from build123d import *

# Parameters (mm, degrees)
SKETCH1_R                 = 3.35
BOSS_EXTRUDE1_DEPTH       = 2.7
SKETCH2_R                 = 2.4
BOSS_EXTRUDE2_DEPTH       = 1.4
SKETCH3_R                 = 1.95
BOSS_EXTRUDE3_DEPTH       = 0.5
F_2_0MM_DOWEL_HOLE1_D     = 2
F_2_0MM_DOWEL_HOLE1_DEPTH = 52.32
F_2_0MM_DOWEL_HOLE1_TIP   = 0.600860619
SKETCH7_W                 = 5.275172559
SKETCH7_H                 = 2.8
BOSS_EXTRUDE4_DEPTH       = 2
F_2_0MM_DOWEL_HOLE2_D     = 1.2
F_2_0MM_DOWEL_HOLE2_DEPTH = 52.32
F_2_0MM_DOWEL_HOLE2_TIP   = 0.360516371
BOSS_EXTRUDE5_DEPTH       = 2.3
BOSS_EXTRUDE6_DEPTH       = 0.5
LPATTERN1_COUNT           = 2
LPATTERN1_PITCH           = 3.5
SKETCH12_R                = 0.5
BOSS_EXTRUDE7_DEPTH       = 1
SKETCH13_W                = 0.512018779
SKETCH13_H                = 0.9
BOSS_EXTRUDE8_DEPTH       = 0.6
BOSS_EXTRUDE9_DEPTH       = 4
SKETCH6_R                 = 2.1
CUT_EXTRUDE1_DEPTH        = 2
SKETCH17_R                = 0.625
CUT_EXTRUDE2_DEPTH        = 2
FILLET1_R                 = 0.1
FILLET2_R                 = 2.7
FILLET3_R                 = 0.5
SKETCH18_R                = 2.8
CUT_EXTRUDE3_DEPTH        = 0.8
BOSS_EXTRUDE10_START      = 0.8
BOSS_EXTRUDE10_DEPTH      = 0.8


with BuildPart() as part:
    # Sketch1 → Boss-Extrude1 (new body)
    with BuildSketch(Plane.XY):
        with Locations(Location((0, 0, 0), (0, 0, 180))):
            Circle(SKETCH1_R)
    extrude(amount=BOSS_EXTRUDE1_DEPTH)

    # Sketch2 → Boss-Extrude2 (add)
    with BuildSketch(Plane.XY.offset(2.7)):
        Circle(SKETCH2_R)
    extrude(amount=BOSS_EXTRUDE2_DEPTH)

    # Sketch3 → Boss-Extrude3 (add)
    with BuildSketch(Plane.XY.offset(4.1)):
        Circle(SKETCH3_R)
    extrude(amount=BOSS_EXTRUDE3_DEPTH)

    # Ø2.0mm Dowel Hole1
    with Locations(Plane.XY.offset(4.6)):
        with Locations((0, 0)):
            Hole(F_2_0MM_DOWEL_HOLE1_D / 2, depth=F_2_0MM_DOWEL_HOLE1_DEPTH)
            with Locations((0, 0, -(F_2_0MM_DOWEL_HOLE1_DEPTH + F_2_0MM_DOWEL_HOLE1_TIP / 2))):  # 118° drill point
                Cone(0, F_2_0MM_DOWEL_HOLE1_D / 2, F_2_0MM_DOWEL_HOLE1_TIP, mode=Mode.SUBTRACT)

    # Sketch7 → Boss-Extrude4 (add)
    with BuildSketch(Plane(origin=(0, 0, 0.4), x_dir=(-1, 0, 0), z_dir=(0, 0, -1))):
        with Locations((4.812413721, 1.05)):
            Rectangle(SKETCH7_W, SKETCH7_H)
    extrude(amount=-BOSS_EXTRUDE4_DEPTH)

    # Ø2.0mm Dowel Hole2
    with Locations(Plane(origin=(0, 0, 0.4), x_dir=(-1, 0, 0), z_dir=(0, 0, -1))):
        with Locations((5.95, 1.35)):
            Hole(F_2_0MM_DOWEL_HOLE2_D / 2, depth=F_2_0MM_DOWEL_HOLE2_DEPTH)
            with Locations((0, 0, -(F_2_0MM_DOWEL_HOLE2_DEPTH + F_2_0MM_DOWEL_HOLE2_TIP / 2))):  # 118° drill point
                Cone(0, F_2_0MM_DOWEL_HOLE2_D / 2, F_2_0MM_DOWEL_HOLE2_TIP, mode=Mode.SUBTRACT)

    # Sketch10 → Boss-Extrude5 (add)
    with BuildSketch(Plane(origin=(0, 0, 0.4), x_dir=(-1, 0, 0), z_dir=(0, 0, -1))):
        with BuildLine():
            Line((0, -3.35), (-4.5, -3.35))
            Line((-4.5, -3.35), (-4.5, -2.796712357))
            Line((-4.5, -2.796712357), (-3.161899091, -1.106749357))
            ThreePointArc((-3.161899091, -1.106749357), (-1.938412966, -2.732225315), (0, -3.35))
        make_face()
    extrude(amount=-BOSS_EXTRUDE5_DEPTH)

    # Sketch11 → Boss-Extrude6 (add)
    with BuildSketch(Plane(origin=(4.5, 0, 0), x_dir=(0, 0, -1), z_dir=(1, 0, 0))):
        with BuildLine():
            Line((-2.7, -3.35), (-2.496243438, -5.634399979))
            ThreePointArc((-2.496243438, -5.634399979), (-1.55, -6.5), (-0.603756562, -5.634399979))
            Line((-0.603756562, -5.634399979), (-0.4, -3.35))
            Line((-0.4, -3.35), (-2.7, -3.35))
        make_face()
    boss_extrude6 = extrude(amount=-BOSS_EXTRUDE6_DEPTH)

    # LPattern1: Boss-Extrude6 ×2
    with Locations(*[(-i * LPATTERN1_PITCH, 0, 0) for i in range(1, LPATTERN1_COUNT)]):
        add(boss_extrude6)

    # Sketch12 → Boss-Extrude7 (add)
    with BuildSketch(Plane.XZ.offset(3.35)):
        with Locations((2.5, 1.575371986)):
            Circle(SKETCH12_R)
    extrude(amount=BOSS_EXTRUDE7_DEPTH)

    # Sketch13 → Boss-Extrude8 (add)
    with BuildSketch(Plane(origin=(0, 0, 1.6), x_dir=(-1, 0, 0), z_dir=(0, 0, -1))):
        with Locations((-3.439131456, 0)):
            Rectangle(SKETCH13_W, SKETCH13_H)
    extrude(amount=-BOSS_EXTRUDE8_DEPTH)

    # Sketch14 → Boss-Extrude9 (add)
    with BuildSketch(Plane(origin=(2.795140845, 0, 0), x_dir=(0, 0, -1), z_dir=(1, 0, 0))):
        Polygon((-0.417568245, 0.970740329), (-0.417568245, 4.082645212), (-3.42580183, 5.903958571), (-6.366262564, 6.498677554), (-6.790223471, 7.512753785), (-8.781855644, 7.695513983), (-7.993219009, 4.904805783), (-4.660696843, 4.230790935), (-2.7, 3.028431634), (-2.7, 0.970740329), align=None)
    extrude(amount=-BOSS_EXTRUDE9_DEPTH)

    # Sketch6 → Cut-Extrude1 (cut)
    with BuildSketch(Plane(origin=(0, 0, 0), x_dir=(-1, 0, 0), z_dir=(0, 0, -1))):
        Circle(SKETCH6_R)
    extrude(amount=-CUT_EXTRUDE1_DEPTH, mode=Mode.SUBTRACT)

    # Sketch17 → Cut-Extrude2 (cut, along a direction that is not the sketch's normal)
    with BuildSketch(Plane(origin=(0, 6.832124657, -0.626943304), x_dir=(1, 0, 0), z_dir=(0, 0.9958160861843439, -0.09138009901775918))):
        with Locations((0.630573116, -8.441313195)):
            Circle(SKETCH17_R)
    extrude(amount=-CUT_EXTRUDE2_DEPTH, dir=(0, 0.962313172469087, 0.2719436671306786), mode=Mode.SUBTRACT)

    # Fillet1
    fillet1_edges = [part.edges().sort_by_distance(p)[0] for p in [
        (2.1, 0, 2),
        (-2.4, 0, 2.7),
        (4, -3.35, 1.55),
        (1, -3.35, 1.55),
        (3.35, 0, 1.6),
        (3.319638535, -0.45, 1.9),
        (3.319638535, 0.45, 1.9),
        (3.35, 0, 2.2),
    ]]
    fillet(fillet1_edges, radius=FILLET1_R)

    # Fillet2
    fillet2_edges = [part.edges().sort_by_distance(p)[0] for p in [
        (-2.284731932, 2.45, 1.4),
    ]]
    fillet(fillet2_edges, radius=FILLET2_R)

    # Fillet3
    # the kernel refuses this fillet: 0.5 mm, written as the material it adds along each edge
    with BuildSketch(Plane(origin=(2.795140845, 3.028431634, 2.7), x_dir=(0, 0.522764913438525, 0.8524768884125898), z_dir=(-1, 0, 0))) as fillet3_piece_1:
        with BuildLine():
            CenterArc((FILLET3_R * 0.559821730124, -FILLET3_R), FILLET3_R, 90, 58.482100164)
            Line((-FILLET3_R * 0.292655158289, -FILLET3_R * 0.477235086561), (0, 0))
            Line((0, 0), (FILLET3_R * 0.559821730124, 0))
        make_face()
    extrude(amount=4)
    with BuildSketch(Plane(origin=(2.795140845, 4.230790935, 4.660696843), x_dir=(0, 0.19823966114604022, 0.9801535781441106), z_dir=(-1, 0, 0))) as fillet3_piece_2:
        with BuildLine():
            CenterArc((FILLET3_R * 0.177081663879, -FILLET3_R), FILLET3_R, 90, 20.083861782)
            Line((-FILLET3_R * 0.166313507063, -FILLET3_R * 0.0608089882382), (0, 0))
            Line((0, 0), (FILLET3_R * 0.177081663879, 0))
        make_face()
    extrude(amount=4)
    with BuildSketch(Plane(origin=(2.795140845, 6.498677554, 6.366262564), x_dir=(0, -0.1982396611460371, -0.9801535781441113), z_dir=(-1, 0, 0))) as fillet3_piece_3:
        with BuildLine():
            CenterArc((FILLET3_R * 0.530337057694, -FILLET3_R), FILLET3_R, 90, 55.877328997)
            Line((-FILLET3_R * 0.297501376428, -FILLET3_R * 0.439033399398), (0, 0))
            Line((0, 0), (FILLET3_R * 0.530337057694, 0))
        make_face()
    extrude(amount=4)
    with BuildSketch(Plane(origin=(2.795140845, 1.846533958, 2.7), x_dir=(0.534296962872843, -0.845296844584703, 0), z_dir=(0, 0, -1))) as fillet3_piece_4:
        with BuildLine():
            CenterArc((0.144932912, -0.49989869), FILLET3_R, 91.153417374, 31.142828348)
            Line((-0.122215569, -0.077250268), (0, 0))
            ThreePointArc((0, 0), (0.067434063, -0.000678778), (0.134868127, 0))
        make_face()
    extrude(amount=2.282431755)
    with BuildSketch(Plane(origin=(-3.33166625, -0.35, 2.4), x_dir=(0.16291161628339781, -0.9866406667474896, 0), z_dir=(0, 0, -1))) as fillet3_piece_5:
        with BuildLine():
            CenterArc((0.42435489, 0.499130817), FILLET3_R, 189.375937442, 77.245195509)
            Line((-0.068965443, 0.417675009), (0, 0))
            ThreePointArc((0, 0), (0.1974429, 0.005823524), (0.394885801, 0))
        make_face()
    extrude(amount=2)
    with BuildSketch(Plane(origin=(0.5, -3.35, 0.4), x_dir=(0, -1, 0), z_dir=(0, 0, 1))) as fillet3_piece_6_section:
        with BuildLine():
            CenterArc((FILLET3_R, -FILLET3_R), FILLET3_R, 90, 90)
            Line((0, -FILLET3_R), (0, 0))
            Line((0, 0), (FILLET3_R, 0))
        make_face()
    fillet3_piece_6 = extrude(amount=2.3, mode=Mode.PRIVATE)
    fillet3_piece_6 = split(fillet3_piece_6, bisect_by=Plane(origin=(0.386269446, -3.56317019, 2.680986331), z_dir=(0, 0.08884208299737703, -0.9960457239949817)), keep=Keep.TOP, mode=Mode.PRIVATE)
    fillet3_piece_6 = split(fillet3_piece_6, bisect_by=Plane(origin=(0.386269446, -3.56317019, 0.419013669), z_dir=(0, 0.08884208299737684, 0.9960457239949817)), keep=Keep.TOP, mode=Mode.PRIVATE)
    add(fillet3_piece_6)
    # the kernel refuses this fillet: 0.5 mm, written as the material it takes off along each edge
    with BuildSketch(Plane(origin=(3.499587338, 4.082645212, 0.417568245), x_dir=(0, 0.5179151427951786, 0.8554319989709583), z_dir=(-1, 0, 0))) as fillet3_2_piece_1:
        with BuildLine():
            CenterArc((FILLET3_R * 0.563557194242, -FILLET3_R), FILLET3_R, 90, 58.807492982)
            Line((-FILLET3_R * 0.291874804729, -FILLET3_R * 0.482084857205), (0, 0))
            Line((0, 0), (FILLET3_R * 0.563557194242, 0))
        make_face()
    extrude(amount=5.408892986, mode=Mode.SUBTRACT)
    with BuildSketch(Plane(origin=(3.557934544, 4.904805783, 7.993219009), x_dir=(0, -0.19823966114603667, -0.9801535781441112), z_dir=(-1, 0, 0))) as fillet3_2_piece_2:
        with BuildLine():
            CenterArc((FILLET3_R * 0.610234959151, -FILLET3_R), FILLET3_R, 90, 62.786002784)
            Line((-FILLET3_R * 0.279069719717, -FILLET3_R * 0.542684804382), (0, 0))
            Line((0, 0), (FILLET3_R * 0.610234959151, 0))
        make_face()
    extrude(amount=5.525587398, mode=Mode.SUBTRACT)
    with BuildSketch(Plane(origin=(3.012833965, 5.903958571, 3.42580183), x_dir=(0, 0.19823966114603944, 0.9801535781441109), z_dir=(-1, 0, 0))) as fillet3_2_piece_3:
        with BuildLine():
            CenterArc((FILLET3_R * 0.174154496328, -FILLET3_R), FILLET3_R, 90, 19.758468965)
            Line((-FILLET3_R * 0.163901334448, -FILLET3_R * 0.0588739429395), (0, 0))
            Line((0, 0), (FILLET3_R * 0.174154496328, 0))
        make_face()
    extrude(amount=4.435386241, mode=Mode.SUBTRACT)

    # Sketch18 → Cut-Extrude3 (cut)
    with BuildSketch(Plane(origin=(0, 0, 0), x_dir=(-1, 0, 0), z_dir=(0, 0, -1))):
        Circle(SKETCH18_R)
    extrude(amount=-CUT_EXTRUDE3_DEPTH, mode=Mode.SUBTRACT)

    # Sketch19 → Boss-Extrude10 (add)
    with BuildSketch(Plane(origin=(0, 0, 0.8), x_dir=(-1, 0, 0), z_dir=(0, 0, -1)).offset(BOSS_EXTRUDE10_START)):
        with BuildLine():
            Line((2.090376166, 0.200817044), (2.787168221, 0.267756059))
            ThreePointArc((2.787168221, 0.267756059), (2.791320225, -0.22029844), (2.710659376, -0.701659282))
            Line((2.710659376, -0.701659282), (2.032994532, -0.526244462))
            ThreePointArc((2.032994532, -0.526244462), (2.093490169, -0.16522383), (2.090376166, 0.200817044))
        make_face()
    extrude(amount=-BOSS_EXTRUDE10_DEPTH)


solid = part.part
Geometry: final body of the model. Coordinates: model frame, mm. A direction names the side the tool comes from. Give positions to 0.01 mm unless a question says otherwise; leave off trailing zeros. Loops run counter-clockwise (first coordinate to the right, second up) from the corner with the lowest first, then second, coordinate; pieces in that order, holes last. Notation, with made-up numbers: (46, 1) - (74, 1) arc R13 ccw to (74, 18) - close; hole circle Ø4 at (-27.75, 41.5). An arc over 180 degrees is marked (long way). One line per question, with ' | ' between items. Start each with the question number.
(1) Pull-direction query (Z, two-part tool) for faces 5 (the flat face through (0.62, 5.68, 7.23)), 6 (the flat face through (2, -3.35, 1)), 7 (the flat face through (0.82, 6.18, 4.79)); classes: released by +Z, released by -Z, zero draft, split by the parting line, or undercut.
(2) Section query A-A on x = -5.95. Return loops of the section in (y, z).
(3) Section query B-B on x = -3. Return loops of the section in (y, z), then the cut area to 3 significant figures.
(4) Reachability of faces 1 (the flat face through (2, -2, 2.7)), 2 (the flat face through (1.5, 1.7, 0.8)), 3 (the flat face through (-6, -0.35, 1)), 4 (the flat face through (0.823, 3.687, 3.773)) from +Z, -Z, +X, -X, +Y, -Y: full face, straight path, thin tool, end or side. Return the list, or none.
(5) Contact query for flat-ended pins moving along their axis: pin 1 (2 mm diameter, centred on x = -1, y = 5, fed in from +Z); pin 2 (1.8 mm diameter, centred on x = 2.5, z = 1.5, fed in from -Y); pin 3 (3 mm diameter, centred on y = 6, z = 5.5, fed in from +X); pin 4 (1 mm diameter, centred on x = -5.95, y = 1.35, fed in from -Z). Output: stop coordinate, or through.
(6) Ray query, line 1 (Y direction, x = 0, z = 0.35); line 2 (X direction, y = 0, z = 0.65); line 3 (X direction, y = 0, z = 1.7). Return the intervals inside material, ascending. Write a range as from..to.
The answers:
1) face 5: undercut | face 6: zero draft | face 7: released by -Z
2) outline: (-0.35, 0.4) - (0.75, 0.4) - (0.75, 2.4) - (-0.35, 2.4) - close; (1.95, 0.4) - (2.45, 0.4) - (2.45, 2.4) - (1.95, 2.4) - close
3) outline: (-1.49, 0) - (1.49, 0) - (1.49, 0.4) - (2.46, 0.4) - (2.46, 2.4) - (1.49, 2.4) - (1.49, 2.7) - (-1.49, 2.7) - close | area: 9.98 mm2
4) face 1: +Z | face 2: -Z | face 3: +Z, -Z, -X, -Y | face 4: +Z, +X, -X
5) pin 1: z = 8.3 | pin 2: y = -4.35 | pin 3: x = 2.8 | pin 4: through
6) line 1: -3.35..-2.8, 2.8..3.35 | line 2: -7.45..-2.1, 2.8..3.35 | line 3: -7.45..-2.1, 2.1..3.7
